```python
from build123d import *

# Parameters (mm, degrees)
BOSS_EXTRUDE1_DEPTH = 5.15
SKETCH2_R           = 1.9675
CUT_EXTRUDE1_DEPTH  = 6.15


with BuildPart() as part:
    # Sketch1 → Boss-Extrude1 (new body)
    with BuildSketch(Plane.XY):
        Polygon((-0.1, -0.1), (3, -0.1), (7, -0.1), (8.1, -0.1), (8.1, 7.1), (-0.1, 7.1), align=None)
    extrude(amount=BOSS_EXTRUDE1_DEPTH)

    # Sketch2 → Cut-Extrude1 (cut, through all)
    with BuildSketch(Plane.XY.offset(5.15)):
        with Locations((4, 4)):
            Circle(SKETCH2_R)
    extrude(amount=-CUT_EXTRUDE1_DEPTH, mode=Mode.SUBTRACT)


solid = part.part
```
Here's how the part is built. I have some questions about the finished solid (model axes, mm). Give positions to 0.01 mm unless a question says otherwise; leave off trailing zeros. Order: outer loops, then holes, each group sorted by start corner. A loop starts at its lowest first (then second) coordinate and runs counter-clockwise, first axis right, second up. Notation, with made-up numbers: M 83,86.5 L 105,86.5 A19 ccw 105,123.5 Z; hole C -34.5,-37 d5. An arc over 180 degrees is marked long. Use a Markdown table: item, result. Add a question column.
1. Suppose I cut it at C-C (z = 4.45). List the corners of the cut face in (x, y) for me (1 decimal), and give its area (3 significant figures).
2. I need wall thicknesses on probe 1 along Y at (x, z) = (4, 2.3); probe 2 along X at (y, z) = (4.5, 2.2); probe 3 along X at (y, z) = (4.25, 0.9). Which ranges of each line are inside material? Lowest first, please. Write a range as from..to.
3. If we mould it in two halves opening along X, with no side actions, what happens to faces 1 (the cylindrical face through (3.57, 2.08, 2.61)), 2 (the flat face through (8.1, 3, 3)), 3 (the flat face through (-0.1, 4, 3))? For each: +X half, -X half, draft (parallel to the pull), parting line (faces both ways), or undercut.
4. Suppose I cut it at A-A (x = 4). List the corners of the cut face in (y, z) for me.
5. Suppose I cut it at B-B (y = 4). List the corners of the cut face in (x, z) for me, and give its area (3 significant figures).
6. For pin 1 Ø2.5 at (x, y) = (4, 4) entering from -Z, with a flat end and sliding along its axis, tell me the tip position at first contact or that it passes through.
Results list:
| question | item | result |
|---|---|---|
| 1 | outline | M -0.1,-0.1 L 8.1,-0.1 L 8.1,7.1 L -0.1,7.1 Z; hole C 4,4 d3.9 |
| 1 | area | 46.9 mm² |
| 2 | probe 1 | y = -0.1..2.03, 5.97..7.1 |
| 2 | probe 2 | x = -0.1..2.1, 5.9..8.1 |
| 2 | probe 3 | x = -0.1..2.05, 5.95..8.1 |
| 3 | face 1 | undercut |
| 3 | face 2 | +X half |
| 3 | face 3 | -X half |
| 4 | outline | M -0.1,0 L 2.03,0 L 2.03,5.15 L -0.1,5.15 Z; M 5.97,0 L 7.1,0 L 7.1,5.15 L 5.97,5.15 Z |
| 5 | outline | M -0.1,0 L 2.03,0 L 2.03,5.15 L -0.1,5.15 Z; M 5.97,0 L 8.1,0 L 8.1,5.15 L 5.97,5.15 Z |
| 5 | area | 22.0 mm² |
| 6 | pin 1 | passes through |
